Build history of the part. All positions in model axes, mm. Face numbers are marked on the shaded views. Coordinates: 2 decimals unless noted, no trailing zeros. Order: outer loops, then holes, each group sorted by start corner. A loop starts at its lowest first (then second) coordinate and runs counter-clockwise, first axis right, second up. Notation, with made-up numbers: (69, -36) - (74, -36) arc R33 ccw to (74, 2) - close; hole circle Ø9 at (-32.75, 61.25). An arc over 180 degrees is marked (long way). Return JSON: item names as keys, results as strings.
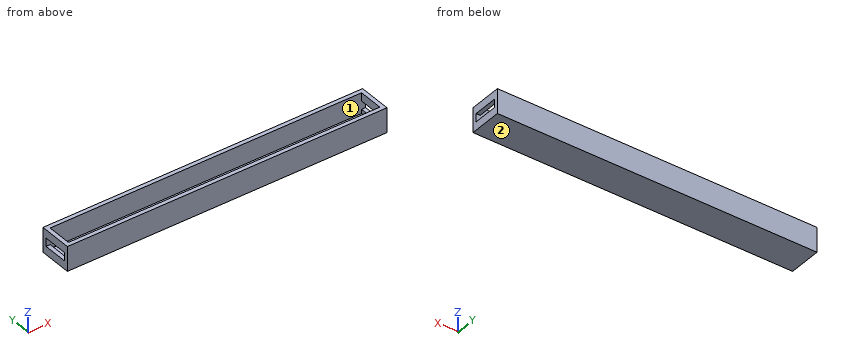
from build123d import *

# Parameters (mm, degrees)
F0_W     = 195
F0_H     = 20
F1_DEPTH = 15
F2_W     = 190
F2_H     = 15
F3_DEPTH = 12.5
F4_W     = 15
F4_H     = 5
F5_DEPTH = 195.001


with BuildPart() as f1:
    # F0 (on Top) → F1 (new body)
    with BuildSketch(Plane.XY):
        Rectangle(F0_W, F0_H)
    extrude(amount=F1_DEPTH)

    # F2 (on face) → F3 (cut)
    with BuildSketch(Plane.XY.offset(15)):
        Rectangle(F2_W, F2_H)
    extrude(amount=-F3_DEPTH, mode=Mode.SUBTRACT)

    # F4 (on face) → F5 (cut, through all)
    with BuildSketch(Plane.YZ.offset(97.5)):
        with Locations((0, 7.5)):
            Rectangle(F4_W, F4_H)
    extrude(amount=-F5_DEPTH, mode=Mode.SUBTRACT)


solid = f1.part
1. Cut at C-C on x = 49. Give the cut face in (y, z), plus the area to 4 significant figures.
Check values:
{"outline": "(-10, 0) - (10, 0) - (10, 15) - (7.5, 15) - (7.5, 2.5) - (-7.5, 2.5) - (-7.5, 15) - (-10, 15) - close", "area": "112.5 mm²"}
2. Cut at A-A on z = 7.75. Give the cut face in (x, y), plus the area to 3 significant figures.
Check values:
{"outline": "(-97.5, -10) - (97.5, -10) - (97.5, -7.5) - (-97.5, -7.5) - close; (-97.5, 7.5) - (97.5, 7.5) - (97.5, 10) - (-97.5, 10) - close", "area": "975 mm²"}
3. Probe L1, parallel to Y at x = 28, z = 14.25; L2, parallel to X at y = -3, z = 10.25; L3, parallel to Z at x = -10, y = -0.5. List the from-to ranges inside material, lowest first.
Check values:
{"L1": "-10 to -7.5, 7.5 to 10", "L2": "-97.5 to -95, 95 to 97.5", "L3": "0 to 2.5"}
4. Mould opens along X. For the marked faces 1 and 2 say: pulls with the +X half, pulls with the -X half, needs draft (parallel to the pull), parting line crosses it, or undercut.
Check values:
{"face 1": "undercut", "face 2": "needs draft"}
5. Cut at B-B on y = 4.25. Give the cut face in (x, z).
Check values:
{"outline": "(-97.5, 0) - (97.5, 0) - (97.5, 5) - (95, 5) - (95, 2.5) - (-95, 2.5) - (-95, 5) - (-97.5, 5) - close; (-97.5, 10) - (-95, 10) - (-95, 15) - (-97.5, 15) - close; (95, 10) - (97.5, 10) - (97.5, 15) - (95, 15) - close"}
6. Drop flat-ended pins along their axis: pin 1 (3 mm diameter, centred on x = 96, y = -2, fed in from -Z); pin 2 (7.5 mm diameter, centred on x = 36, y = -3.5, fed in from +Z). Give the stop position or say it passes through.
Check values:
{"pin 1": "z = 0", "pin 2": "z = 2.5"}
